Could you check a few things on this model? Use its own coordinates, in mm. A direction names the side the tool comes from. Coordinates: 2 decimals unless noted, no trailing zeros. Write each loop counter-clockwise with the first axis right and the second up, starting at its lowest first coordinate (ties: lowest second). Pieces come first, ordered by that corner, then holes.
Item 1: I want a section at C-C on z = -6.5. Please give me the cut outline in (x, y) (3 decimals), then the cut area to 3 significant figures.
Item 2: Which directions (+Z, -Z, +X, -X, +Y, -Y) give clear straight access to the entire face, cutting with the end or side of a thin tool? Please do faces 1 (the cylindrical face through (43.12, -14.77, -26.86)), 2 (the flat face through (20.173, -14.774, -39.509)), 3 (the cylindrical face through (32.88, -14.77, -19.25)), 4 (the cylindrical face through (-32.84, 7.56, -19.32)), 5 (the flat face through (20.173, 7.55, -39.509)).
Item 3: For P1, Ø3, axis at y = -18.5, z = -34.5, coming from the +X side; P2, Ø4, axis at x = 18.5, y = -0.5, coming from the -Z side; P3, Ø6, axis at y = -17, z = 34.5, coming from the -X side, each with a flat end and sliding along its axis, tell me the tip position at first contact or that it passes through.
Item 4: I want a section at B-B on y = -19.5. Please give me the cut outline in (x, z), then the cut area to 3 significant figures.
Item 5: If I drill on probe 1 along Z at (x, y) = (0, 3) (3 decimals); probe 2 along Y at (x, z) = (21, -15.5); probe 3 along Z at (x, y) = (-22, -15), over which ranges is the centre line in solid material (lowest first)?
Item 6: Thinking about a two-plate mould opening in X: for faces 6 (the cylindrical face through (-0.3, -14.6, 38.1)), 7 (the cylindrical face through (-57.095, -0.1, 2.513)), 8 (the cylindrical face through (43.12, 7.55, -26.86)), which applies, +X half, -X half, draft (parallel to the pull), parting line (faces both ways), or undercut?
Item 7: I want a section at D-D on z = -22. Please give me the cut outline in (x, y) (3 decimals), then the cut area to 3 significant figures.
Item 8: I want a section at A-A on x = 0. Please give me the cut outline in (y, z) (3 decimals), then the cut area to 3 significant figures.
from build123d import *

# Parameters (mm, degrees)
F0_R     = 57.15
F0_R_2   = 15.875
F1_DEPTH = 7.112
F3_DEPTH = 15.113
F2_R     = 7.112
F4_DEPTH = 15.114


with BuildPart() as f1:
    # F0 (on Front) → F1 (new body, symmetric)
    with BuildSketch(Plane.XZ):
        Circle(F0_R)
        Circle(F0_R_2, mode=Mode.SUBTRACT)
    extrude(amount=F1_DEPTH, both=True)

    # F2 (on face) → F3 (join, symmetric)
    with BuildSketch(Plane.XZ.offset(7.112)):
        with BuildLine():
            ThreePointArc((-17.325537, -33.932813), (-32.995568, -19.05), (-38.049446, 1.962051))
            Line((-38.049446, 1.962051), (-50.732595, 2.616068))
            ThreePointArc((-50.732595, 2.616068), (-43.994091, -25.4), (-23.100716, -45.24375))
            Line((-23.100716, -45.24375), (-17.325537, -33.932813))
        make_face()
        with BuildLine():
            ThreePointArc((27.631879, 42.627682), (0, 50.8), (-27.631879, 42.627682))
            Line((-27.631879, 42.627682), (-20.723909, 31.970762))
            ThreePointArc((-20.723909, 31.970762), (0, 38.1), (20.723909, 31.970762))
            Line((20.723909, 31.970762), (27.631879, 42.627682))
        make_face()
        with BuildLine():
            Line((17.325537, -33.932813), (23.100716, -45.24375))
            ThreePointArc((23.100716, -45.24375), (43.32526, -26.52474), (50.8, 0))
            ThreePointArc((50.8, 0), (50.796375, 0.606886), (50.7855, 1.213686))
            Line((50.7855, 1.213686), (38.089125, 0.910265))
            ThreePointArc((38.089125, 0.910265), (32.729286, -19.503943), (17.325537, -33.932813))
        make_face()
    extrude(amount=F3_DEPTH, both=True)

    # F2 (on face) → F4 (cut, through all)
    with BuildSketch(Plane.XZ.offset(7.112)):
        with Locations((-31.675745, 18.288)):
            Circle(F2_R)
        with Locations((31.675745, 18.288)):
            Circle(F2_R)
        with Locations((0, -36.576)):
            Circle(F2_R)
    extrude(amount=-F4_DEPTH, mode=Mode.SUBTRACT)


solid = f1.part
Response values:
1. outline: (-56.779, -7.112) - (-50.382, -7.112) - (-50.382, -22.225) - (-37.541, -22.225) - (-37.541, -7.112) - (-14.483, -7.112) - (-14.483, 7.112) - (-37.541, 7.112) - (-37.541, 8.001) - (-50.382, 8.001) - (-50.382, 7.112) - (-56.779, 7.112) - close; (14.483, -7.112) - (37.541, -7.112) - (37.541, -22.225) - (50.382, -22.225) - (50.382, -7.112) - (56.779, -7.112) - (56.779, 7.112) - (50.382, 7.112) - (50.382, 8.001) - (37.541, 8.001) - (37.541, 7.112) - (14.483, 7.112) - close
1. area: 1,610 mm2
2. face 1: -Z, +X, -Y
2. face 2: -Z, -Y
2. face 3: -Y
2. face 4: +Y
2. face 5: -Z, +Y
3. P1: stops at x = 38.62
3. P2: stops at z = -54.72
3. P3: stops at x = -24.31
4. outline: (-50.73, 2.62) arc R50.8 ccw to (-23.1, -45.24) - (-17.33, -33.93) arc R38.1 cw to (-38.05, 1.96) - close; (-27.63, 42.63) - (-20.72, 31.97) arc R38.1 cw to (20.72, 31.97) - (27.63, 42.63) arc R50.8 ccw to start; (17.33, -33.93) - (23.1, -45.24) arc R50.8 ccw to (50.8, 0) arc R50.8 ccw to (50.79, 1.21) - (38.09, 0.91) arc R38.1 cw to start
4. area: 1,930 mm2
5. probe 1: z = -57.15 to -43.688, -29.464 to -15.875, 15.875 to 57.15
5. probe 2: y = -7.11 to 7.11
5. probe 3: z = -43.09 to -31.11, 33.94 to 45.79
6. face 6: undercut
6. face 7: parting line
6. face 8: +X half
7. outline: (-52.746, -7.112) - (-45.789, -7.112) - (-45.789, -22.225) - (-31.106, -22.225) - (-31.106, -7.112) - (31.106, -7.112) - (31.106, -22.225) - (45.789, -22.225) - (45.789, -7.112) - (52.746, -7.112) - (52.746, 7.112) - (45.789, 7.112) - (45.789, 8.001) - (31.106, 8.001) - (31.106, 7.112) - (-31.106, 7.112) - (-31.106, 8.001) - (-45.789, 8.001) - (-45.789, 7.112) - (-52.746, 7.112) - close
7. area: 1,970 mm2
8. outline: (-22.225, 38.1) - (-7.112, 38.1) - (-7.112, 15.875) - (7.112, 15.875) - (7.112, 38.1) - (8.001, 38.1) - (8.001, 50.8) - (7.112, 50.8) - (7.112, 57.15) - (-7.112, 57.15) - (-7.112, 50.8) - (-22.225, 50.8) - close; (-7.112, -57.15) - (7.112, -57.15) - (7.112, -43.688) - (-7.112, -43.688) - close; (-7.112, -29.464) - (7.112, -29.464) - (7.112, -15.875) - (-7.112, -15.875) - close
8. area: 1,180 mm2
